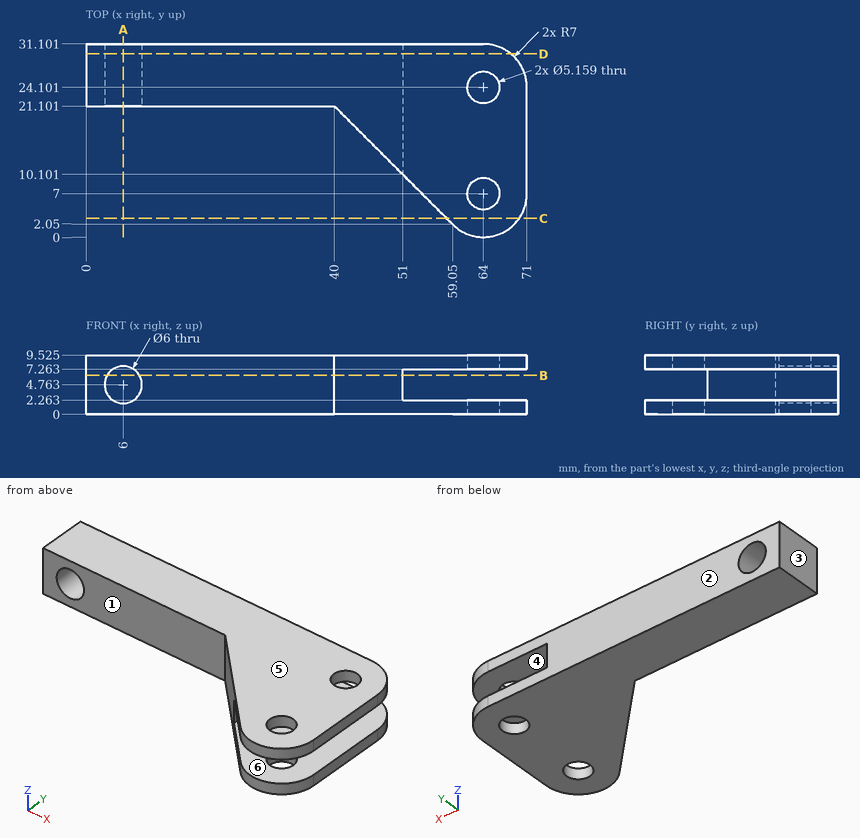
The figure shows three views and two pictorial views of one solid part (mm, origin at its lowest corner). Answer the questions. A direction names the side the tool comes from. Round coordinates to 2 decimals unless told otherwise and drop trailing zeros. Write each loop counter-clockwise with the first axis right and the second up, starting at its lowest first coordinate (ties: lowest second). Pieces come first, ordered by that corner, then holes. Notation, with made-up numbers: M -2.5,23 L 11.5,23 A11 ccw 11.5,30 Z; hole C 8.5,20 d9. An arc over 180 degrees is marked long. Use a Markdown table: item, result.
1) Determine the mould class of the marked faces 3, 4, 5 and 6 for opening direction Z: pulls with the +Z half, pulls with the -Z half, needs draft (parallel to the pull), parting line crosses it, or undercut.
Taken from the geometry:
| item | result |
|---|---|
| face 3 | needs draft |
| face 4 | undercut |
| face 5 | pulls with the +Z half |
| face 6 | undercut |
2) Consider line 1 (Y direction, x = 64, z = 8); line 2 (X direction, y = 24, z = 4.5); line 3 (Z direction, x = 59.5, y = 10.5) (1 decimal). Determine where each line is inside the solid, lowest interval first. Write a range as [from, to].
Taken from the geometry:
| item | result |
|---|---|
| line 1 | y = [0, 4.42], [9.58, 21.52], [26.68, 31.1] |
| line 2 | x = [0, 3.01], [8.99, 51] |
| line 3 | z = [0, 2.3], [7.3, 9.5] |
3) Flat-ended cylindrical pins translate along their axes: pin 1 (6 mm diameter, centred on x = 64, y = 24.1, fed in from +Z) (1 decimal); pin 2 (2 mm diameter, centred on y = 19.5, z = 3, fed in from -X); pin 3 (2.5 mm diameter, centred on y = 15.5, z = 5.5, fed in from +X); pin 4 (5 mm diameter, centred on x = 29.5, z = 2.5, fed in from -Y). Find the tip coordinate at first contact, or state that the pin passes through.
Taken from the geometry:
| item | result |
|---|---|
| pin 1 | stops at z = 9.5 |
| pin 2 | stops at x = 40.6 |
| pin 3 | stops at x = 51 |
| pin 4 | stops at y = 21.1 |
4) The part is cut by section C-C on y = 3. Give the vertices of the cut face in (x, z) (1 decimal).
Taken from the geometry:
| item | result |
|---|---|
| outline | M 58.1,0 L 69.7,0 L 69.7,2.3 L 58.1,2.3 Z; M 58.1,7.3 L 69.7,7.3 L 69.7,9.5 L 58.1,9.5 Z |
5) Which of the six approach directions +Z, -Z, +X, -X, +Y, -Y give full straight-line access (tool end or side, diameter ignored) to the marked faces 1 and 2?
Taken from the geometry:
| item | result |
|---|---|
| face 1 | +Z, -Z, -X, -Y |
| face 2 | +Z, -Z, +X, -X, +Y |
6) The part is cut by section B-B on z = 6.25. Give the vertices of the cut face in (x, y) (1 decimal).
Taken from the geometry:
| item | result |
|---|---|
| outline | M 0,21.1 L 3.4,21.1 L 3.4,31.1 L 0,31.1 Z; M 8.6,21.1 L 40,21.1 L 51,10.1 L 51,31.1 L 8.6,31.1 Z |
7) The part is cut by section D-D on y = 29.5. Give the vertices of the cut face in (x, z) (1 decimal).
Taken from the geometry:
| item | result |
|---|---|
| outline | M 0,0 L 68.5,0 L 68.5,2.3 L 51,2.3 L 51,7.3 L 68.5,7.3 L 68.5,9.5 L 0,9.5 Z; hole C 6,4.8 d6 |
8) The part is cut by section A-A on x = 6. Give the vertices of the cut face in (y, z) (1 decimal).
Taken from the geometry:
| item | result |
|---|---|
| outline | M 21.1,0 L 31.1,0 L 31.1,1.8 L 21.1,1.8 Z; M 21.1,7.8 L 31.1,7.8 L 31.1,9.5 L 21.1,9.5 Z |
